Could you check a few things on this model? Use its own coordinates, in mm. A direction names the side the tool comes from. Give positions to 0.01 mm unless a question says otherwise; leave off trailing zeros. Loops run counter-clockwise (first coordinate to the right, second up) from the corner with the lowest first, then second, coordinate; pieces in that order, holes last. Notation, with made-up numbers: (-14.5, 22.5) - (26.5, 22.5) arc R29 ccw to (26.5, 59.5) - close; hole circle Ø4 at (46.5, 7.25). An arc over 180 degrees is marked (long way). Use CSV: the item, a comma, the result in double quotes.
from build123d import *

# Parameters (mm, degrees)
SKETCH_1_R          = 3.2500000000000004
SKETCH_1_R_2        = 8.149999999999999
EXTRUDE_1_DEPTH     = 4
SKETCH_1_3_R        = 11.999999999999993
SKETCH_1_3_R_2      = 8.149999999999999
SKETCH_1_3_R_3      = 9.500000000000002
EXTRUDE_2_DEPTH     = 23.15
EXTRUDE_START       = 9
SKETCH_1_4_R        = 8.149999999999999
SKETCH_1_4_R_2      = 5.999999999999998
EXTRUDE_3_DEPTH     = 8
EXTRUDE_4_DEPTH     = 9.000000000000002
FILLET_1_R          = 2
EXTRUDE_5_DEPTH     = 27
FILLET_2_R          = 1
SKETCH_1_6_R        = 9.500000000000002
SKETCH_1_6_R_2      = 8.149999999999999
CUT_EXTRUDE_1_DEPTH = 2
CHAMFER_1_SIZE      = 2.3
CHAMFER_2_SIZE      = 1.3
FILLET_4_R          = 3.5
SKETCH_1_7_R        = 3.2500000000000004
EXTRUDE_6_DEPTH     = 5.4
FILLET_3_R          = 1
CHAMFER_3_SIZE      = 0.5


with BuildPart() as part:
    # Эскиз1 → Бобышка-Вытянуть1 (new body)
    with BuildSketch(Plane.XY):
        with BuildLine():
            Line((-14.999999999999972, -8.963730931198981), (20.850000000000577, -8.96373093119897))
            ThreePointArc((20.85000000000058, -8.963730931198967), (32.70050757538239, 1.1480237971749345), (24.57944414926456, 14.44202403449797))
            Line((24.57944414926456, 14.44202403449797), (-11.068586896529624, 26.098187192163547))
            ThreePointArc((-11.068586896529625, 26.098187192163547), (-20.788047002520305, 25.117990405859814), (-25.455246310980815, 16.536269068801015))
            Line((-25.455246310980815, 16.536269068801015), (-25.45524631098081, 1.4915153797818874))
            ThreePointArc((-25.45524631098081, 1.4915153797818874), (-22.392975565470174, -5.9014601856883235), (-14.999999999999972, -8.96373093119898))
        make_face()
        Polygon((-10.849999999999971, 7.491515379781886), (-19.149999999999974, 7.491515379781886), (-19.149999999999974, 22.491515379781884), (-10.849999999999973, 22.491515379781884), align=None, mode=Mode.SUBTRACT)
        with Locations((-14.999999999999972, 1.4915153797818852)):
            Circle(SKETCH_1_R, mode=Mode.SUBTRACT)
        with Locations((20.85000000000058, 3.036269068801026)):
            Circle(SKETCH_1_R_2, mode=Mode.SUBTRACT)
    extrude(amount=EXTRUDE_1_DEPTH)

    # Эскиз1<3> → Бобышка-Вытянуть2 (add)
    # profile 1 of 3: a face of its own
    with BuildSketch(Plane.XY):
        with BuildLine():
            Line((-0.29999999999996874, -8.96373093119897), (20.85000000000058, -8.96373093119897))
            ThreePointArc((20.850000000000577, -8.963730931198967), (8.999492424618776, 4.924514340427118), (24.57944414926456, 14.44202403449797))
            Line((24.57944414926456, 14.442024034497972), (-0.2999999999999723, 22.57708372133782))
            Line((-0.2999999999999722, 22.57708372133782), (-0.2999999999999704, -8.96373093119897))
        make_face()
    # profile 2 of 3: a face of its own
    with BuildSketch(Plane.XY):
        with Locations((20.85000000000058, 3.036269068801026)):
            Circle(SKETCH_1_3_R)
        with Locations((20.85000000000058, 3.036269068801026)):
            Circle(SKETCH_1_3_R_2, mode=Mode.SUBTRACT)
    # profile 3 of 3: a face of its own
    with BuildSketch(Plane.XY):
        with Locations((20.85000000000058, 3.036269068801026)):
            Circle(SKETCH_1_3_R_3)
        with Locations((20.85000000000058, 3.036269068801026)):
            Circle(SKETCH_1_3_R_2, mode=Mode.SUBTRACT)
    extrude(amount=EXTRUDE_2_DEPTH)

    # Эскиз1<4> → Бобышка-Вытянуть3 (add)
    with BuildSketch(Plane.XY.offset(EXTRUDE_START)):
        with Locations((20.85000000000058, 3.036269068801026)):
            Circle(SKETCH_1_4_R)
        with Locations((20.85000000000058, 3.036269068801026)):
            Circle(SKETCH_1_4_R_2, mode=Mode.SUBTRACT)
    extrude(amount=EXTRUDE_3_DEPTH)

    # Эскиз1<5> → Бобышка-Вытянуть4 (add)
    with BuildSketch(Plane.XY):
        Polygon((-10.849999999999971, 7.491515379781886), (-10.849999999999973, 22.491515379781884), (-19.149999999999974, 22.491515379781884), (-19.149999999999974, 7.491515379781886), align=None)
    extrude(amount=EXTRUDE_4_DEPTH)

    # Скругление1
    fillet_1_edges = [part.edges().sort_by_distance(p)[0] for p in [
        (-0.29999999999997223, 22.57708372133782, 13.575),
    ]]
    fillet(fillet_1_edges, radius=FILLET_1_R)

    # Эскиз4 → Бобышка-Вытянуть5 (add)
    with BuildSketch(Plane.XZ.offset(8.96373093119897)):
        Polygon((-4.879999999999971, 26.15), (-4.87999999999997, 21.15), (-0.2999999999999704, 14.85), (-0.2999999999999704, 23.150000000000002), (-1.8799999999999704, 23.150000000000002), (-1.8799999999999704, 26.15), align=None)
    extrude(amount=-EXTRUDE_5_DEPTH)

    # Скругление2
    fillet_2_edges = [part.edges().sort_by_distance(p)[0] for p in [
        (-0.29999999999996957, -8.96373093119897, 9.425),
        (-2.589999999999968, 18.03626906880103, 18),
        (-4.879999999999969, 18.03626906880103, 23.65),
        (-1.8799999999999681, 18.03626906880103, 24.65),
        (-2.58999999999997, -8.96373093119897, 18),
        (-1.8799999999999704, -8.96373093119897, 24.65),
        (-4.879999999999971, -8.96373093119897, 23.65),
    ]]
    fillet(fillet_2_edges, radius=FILLET_2_R)

    # Эскиз1<6> → Вырез-Вытянуть1 (cut)
    with BuildSketch(Plane.XY):
        with Locations((20.85000000000058, 3.036269068801026)):
            Circle(SKETCH_1_6_R)
        with Locations((20.85000000000058, 3.036269068801026)):
            Circle(SKETCH_1_6_R_2, mode=Mode.SUBTRACT)
    extrude(amount=CUT_EXTRUDE_1_DEPTH, mode=Mode.SUBTRACT)

    # Фаска1
    # the kernel refuses this chamfer: 2.3 mm, written as the material it takes off along each edge
    with BuildSketch(Plane(origin=(20.85000000000058, 3.036269068801026, 9), x_dir=(1, 0, 0), z_dir=(0, -1, 0))) as chamfer_1_piece_1_section:
        Polygon((5.9999999999999964, CHAMFER_1_SIZE), (5.9999999999999964 + CHAMFER_1_SIZE, 0), (5.9999999999999964, 0), align=None)
    chamfer_1_piece_1 = revolve(axis=Axis((20.85000000000058, 3.036269068801026, 9), (0, 0, 1)), mode=Mode.PRIVATE)
    chamfer_1_piece_1 = chamfer_1_piece_1 & Plane(origin=(20.85000000000058, 3.036269068801026, 10.222457747954977), x_dir=(1, 0, 0), z_dir=(0, 0, -1)) * Cylinder(8.149999999999999, 34, mode=Mode.PRIVATE)
    add(chamfer_1_piece_1, mode=Mode.SUBTRACT)

    # Фаска2
    chamfer_2_edges = [part.edges().sort_by_distance(p)[0] for p in [
        (12.700000000000582, 3.036269068801027, 2),
    ]]
    chamfer(chamfer_2_edges, length=CHAMFER_2_SIZE)

    # Скругление4
    # the kernel refuses this fillet: 3.5 mm, written as the material it adds along each edge
    with BuildSketch(Plane(origin=(0.7000000000000293, -7.963730931198976, 4), x_dir=(-0.9999802608561372, 0.006283143965558403, 0), z_dir=(-0.006283143965558403, -0.9999802608561372, 0))) as fillet_4_piece_1_section:
        with BuildLine():
            CenterArc((-0.9999999999999992 - FILLET_4_R, -FILLET_4_R), FILLET_4_R, 0, 90)
            Line((-0.9999999999999979, -FILLET_4_R), (-0.9999999999999992, 0))
            Line((-0.9999999999999992, 0), (-0.9999999999999992 - FILLET_4_R, 0))
        make_face()
    fillet_4_piece_1 = revolve(axis=Axis((0.7000000000000293, -7.963730931198976, 4), (0, 0, -1)), revolution_arc=359.64000000000004, mode=Mode.PRIVATE)
    fillet_4_piece_1 = split(fillet_4_piece_1, bisect_by=Plane(origin=(-0.06522476751896455, -8.963730931198977, 5.353005928395178), z_dir=(-3e-16, 1, 0)), keep=Keep.TOP, mode=Mode.PRIVATE)
    add(fillet_4_piece_1)
    with BuildSketch(Plane(origin=(-0.2999999999999705, -7.963730931198976, 4), x_dir=(-1, -6e-17, 0), z_dir=(-6e-17, 1, 0))) as fillet_4_piece_2:
        with BuildLine():
            CenterArc((FILLET_4_R, FILLET_4_R), FILLET_4_R, 180, 90)
            Line((-4.4e-16, FILLET_4_R), (0, 0))
            Line((0, 0), (FILLET_4_R, 0))
        make_face()
    extrude(amount=27.782655425625357)
    with BuildSketch(Plane(origin=(1.7000000000000277, 19.818924494426383, 4), x_dir=(-0.9998226837850567, -0.018830852047809543, 0), z_dir=(-0.018830852047809543, 0.9998226837850567, 0))) as fillet_4_piece_3_section:
        with BuildLine():
            CenterArc((-2.000000000000004 - FILLET_4_R, FILLET_4_R), FILLET_4_R, 270, 90)
            Line((-2.000000000000004, FILLET_4_R), (-2.000000000000004, 0))
            Line((-2.000000000000004, 0), (-2.000000000000004 - FILLET_4_R, 0))
        make_face()
    fillet_4_piece_3 = revolve(axis=Axis((1.7000000000000277, 19.818924494426383, 4), (0, 0, 1)), revolution_arc=358.921007878005, mode=Mode.PRIVATE)
    fillet_4_piece_3 = split(fillet_4_piece_3, bisect_by=Plane(origin=(0.6026329252520348, 22.28194156791278, 5.095559189965934), z_dir=(-0.3107870124386654, -0.950479580474746, 0)), keep=Keep.TOP, mode=Mode.PRIVATE)
    add(fillet_4_piece_3)

    # Эскиз1<7> → Бобышка-Вытянуть6 (add)
    with BuildSketch(Plane.XY):
        Polygon((-10.849999999999971, 7.491515379781886), (-19.149999999999974, 7.491515379781886), (-19.149999999999974, -4.508484620218114), (-10.849999999999971, -4.508484620218115), align=None)
        with Locations((-14.999999999999972, 1.4915153797818852)):
            Circle(SKETCH_1_7_R, mode=Mode.SUBTRACT)
    extrude(amount=EXTRUDE_6_DEPTH)

    # Скругление3
    fillet_3_edges = [part.edges().sort_by_distance(p)[0] for p in [
        (-19.149999999999974, -4.508484620218114, 4.7),
        (-10.849999999999971, -4.508484620218114, 4.7),
        (-19.149999999999974, 22.491515379781884, 6.500000000000001),
        (-19.149999999999974, 7.491515379781886, 7.200000000000001),
        (-10.849999999999971, 7.491515379781886, 7.200000000000001),
        (-10.849999999999973, 22.491515379781884, 6.500000000000001),
    ]]
    fillet(fillet_3_edges, radius=FILLET_3_R)

    # Фаска3
    chamfer_3_edges = [part.edges().sort_by_distance(p)[0] for p in [
        (11.350000000000579, 3.0362690688010274, 0),
        (12.700000000000582, 3.036269068801027, 23.15),
    ]]
    chamfer(chamfer_3_edges, length=CHAMFER_3_SIZE)


solid = part.part
1) I'm going to push flat-ended pins straight in: P1, Ø6, axis at x = -8, y = 1.5, coming from the -Z side; P2, Ø12, axis at y = 17.5, z = 21.5, coming from the +X side; P3, Ø1.8, axis at x = -2.5, z = 22.5, coming from the +Y side; P4, Ø5.5, axis at y = 10.5, z = 7.5, coming from the -X side. Where does each tip first touch, or does it pass through?
Answer below:
P1,"stops at z = 0"
P2,"stops at x = 29.36"
P3,"stops at y = 18.04"
P4,"stops at x = -19.15"
2) We'd pull the mould along X, two halves only. Please class faces 5 (the flat face through (-4.88, 4, 24)), 6 (the conical face through (15.982, -0.696, 11.166)), 7 (the flat face through (10.97, 18.89, 11.41)): +X half, -X half, draft (parallel to the pull), parting line (faces both ways), or undercut.
Answer below:
face 5,"-X half"
face 6,"undercut"
face 7,"+X half"
3) Suppose I cut it at A-A (z = 4.75). Please give me the cut outline in (x, y), plus the area to 3 significant figures.
Answer below:
outline,"(-19.15, -3.51) arc R1 ccw to (-18.15, -4.51) - (-11.85, -4.51) arc R1 ccw to (-10.85, -3.51) - (-10.85, 21.49) arc R1 ccw to (-11.85, 22.49) - (-18.15, 22.49) arc R1 ccw to (-19.15, 21.49) - close; (-1.63, -7.96) arc R2.33 ccw to (-1.41, -8.96) - (20.85, -8.96) arc R12 ccw to (24.58, 14.44) - (-0.21, 22.55) arc R3.33 ccw to (-1.63, 19.82) - close; hole circle Ø6.5 at (-15, 1.49); hole circle Ø16.3 at (20.85, 3.04)"
area,"843 mm2"
4) Suppose I cut it at B-B (z = 12.5). Please give me the cut outline in (x, y), plus the area to 3 significant figures.
Answer below:
outline,"(-0.3, -7.96) arc R1 ccw to (0.7, -8.96) - (20.85, -8.96) arc R12 ccw to (24.58, 14.44) - (2.32, 21.72) arc R2 ccw to (-0.3, 19.82) - close; hole circle Ø12 at (20.85, 3.04)"
area,"706 mm2"
5) Suppose I cut it at C-C (y = 15.5). Please give me the cut outline in (x, z), plus the area to 3 significant figures.
Answer below:
outline,"(-25.46, 0) - (21.34, 0) - (21.34, 23.15) - (-1.88, 23.15) - (-1.88, 26.15) - (-4.88, 26.15) - (-4.88, 21.15) - (-0.3, 14.85) - (-0.3, 7.5) arc R3.5 cw to (-3.8, 4) - (-10.85, 4) - (-10.85, 9) - (-19.15, 9) - (-19.15, 4) - (-25.46, 4) - close"
area,"678 mm2"
6) Which directions (+Z, -Z, +X, -X, +Y, -Y) give clear straight access to the entire face, cutting with the end or side of a thin tool? Please do faces 1 (the cylindrical face through (0.547, 21.453, 15.435)), 2 (the flat face through (-2, 18.036, 21)), 3 (the cylindrical face through (-1.3, 5.73, 5.05)), 4 (the flat face through (-19.15, 12, 6)).
Answer below:
face 1,"+Z, +Y"
face 2,"+Z, -X, +Y"
face 3,"+Y, -Y"
face 4,"+Z, -X, +Y, -Y"
7) I need wall thicknesses on line 1 along X through (y, z) = (3.5, 9); line 2 along Z through (x, y) = (10.5, 16); line 3 along Z through (x, y) = (-11, -3.5). Which ranges of each line are inside material? Lowest first, please.
Answer below:
line 1,"x = -0.3 to 12.71, 28.99 to 32.84"
line 2,"z = 0 to 23.15"
line 3,"z = 0 to 5.4"
8) Suppose I cut it at D-D (x = 5). Please give me the cut outline in (y, z), plus the area to 3 significant figures.
Answer below:
outline,"(-8.96, 0) - (20.84, 0) - (20.84, 23.15) - (-8.96, 23.15) - close"
area,"690 mm2"
